from build123d import *

# Parameters (mm, degrees)
SKETCH_1_R          = 4.9999999999999964
EXTRUDE_1_DEPTH     = 18
SKETCH_2_R          = 5
EXTRUDE_2_DEPTH     = 8
FILLET_2_R          = 2
EXTRUDE_4_DEPTH     = 11.3
SKETCH_8_W          = 3.000000000000001
SKETCH_8_H          = 6.0000000000000036
CUT_EXTRUDE_3_DEPTH = 20
SKETCH_9_R          = 2.250000000000002
CUT_EXTRUDE_4_DEPTH = 78.37023084919184
FILLET_1_R          = 1
EXTRUDE_5_DEPTH     = 8
FILLET_3_R          = 2
EXTRUDE_6_DEPTH     = 11.3
FILLET_4_R          = 0.7
CHAMFER_2_SIZE      = 0.7
CUT_EXTRUDE_5_REACH = 123.985
CUT_EXTRUDE_6_DEPTH = 96.67513972142032


# Read off the part's stored shape, not the designer's step: 镜向1
with BuildPart() as part:
    # 草图1 → 凸台-拉伸1 (new body)
    with BuildSketch(Plane.XY):
        with BuildLine():
            Line((61.00000000000003, -13.176914536239765), (43, 17.999999999999996))
            Line((43, 17.999999999999996), (0, 18))
            ThreePointArc((0, 18), (-18, 2.2e-15), (0, -18))
            Line((0, -18), (43, -17.999999999999996))
            ThreePointArc((43, -17.999999999999996), (52.31748562369077, -16.77332974640645), (61.00000000000003, -13.176914536239765))
        make_face()
        with Locations((29.77, 0)):
            Circle(SKETCH_1_R, mode=Mode.SUBTRACT)
    extrude(amount=EXTRUDE_1_DEPTH)

    # 草图2 → 凸台-拉伸2 (add)
    with BuildSketch(Plane.XY.offset(18)):
        with BuildLine():
            Line((8.951308150188659, -4.435), (20.807256279464415, -4.435))
            ThreePointArc((20.807256279464415, -4.434999999999999), (19.769999999999996, 4.4e-16), (20.807256279464415, 4.435))
            Line((20.807256279464415, 4.435), (8.951308150188659, 4.435))
            ThreePointArc((8.951308150188659, 4.434999999999999), (9.989751878782268, -6.7e-16), (8.951308150188659, -4.435))
        make_face()
        Circle(SKETCH_2_R)
    extrude(amount=EXTRUDE_2_DEPTH)

    # 圆角2
    fillet_2_edges = [part.edges().sort_by_distance(p)[0] for p in [
        (20.807256279464415, -4.434999999999999, 22),
        (20.807256279464415, 4.434999999999999, 22),
        (8.951308150188659, 4.434999999999999, 22),
        (8.951308150188659, -4.434999999999999, 22),
    ]]
    fillet(fillet_2_edges, radius=FILLET_2_R)

    # 草图7 → 凸台-拉伸4 (add)
    with BuildSketch(Plane(origin=(33.99999999999993, 33.588457268120045, 0), x_dir=(0, 0, -1), z_dir=(-0.866025403784438, -0.5000000000000009, 0))):
        Polygon((-5.599999999999984, 54.00000000000014), (-12.400000000000015, 54.00000000000014), (-12.400000000000004, 18.00000000000018), (-5.599999999999972, 18.00000000000019), align=None)
        Polygon((-2.9999999999999973, 33.70000000000016), (-1.041e-14, 33.70000000000016), (-1.041e-14, 38.30000000000017), (-2.9999999999999956, 38.30000000000017), align=None)
        Polygon((-15.000000000000004, 38.30000000000017), (-17.99999999999999, 38.30000000000017), (-17.99999999999999, 33.70000000000016), (-15.000000000000002, 33.70000000000016), align=None)
    extrude(amount=-EXTRUDE_4_DEPTH)

    # 草图8 → 切除-拉伸3 (cut)
    with BuildSketch(Plane(origin=(49.8303156968241, 28.769546181365495, -2.936e-14), x_dir=(-5.4e-16, -3.2e-16, 1), z_dir=(0.866025403784438, 0.500000000000001, 0))):
        with Locations((8.99999999999995, 23.911542731880154)):
            Rectangle(SKETCH_8_W, SKETCH_8_H)
    extrude(amount=-CUT_EXTRUDE_3_DEPTH, mode=Mode.SUBTRACT)

    # 草图9 → 切除-拉伸4 (cut, through all)
    with BuildSketch(Plane(origin=(-8.8e-16, 1.52e-15, 5.59999999999997), x_dir=(-1, 0, -1e-16), z_dir=(1e-16, -1.7e-16, -1))):
        with Locations(Location((-60.946152422706646, -1.0836477965031495, 0), (0, 0, 90))):
            Circle(SKETCH_9_R)
        with Locations(Location((-53.44615242270663, 11.90673326026341, 0), (0, 0, 90))):
            Circle(SKETCH_9_R)
    extrude(amount=-CUT_EXTRUDE_4_DEPTH, mode=Mode.SUBTRACT)

    # 圆角1
    fillet_1_edges = [part.edges().sort_by_distance(p)[0] for p in [
        (54.62583302491982, 0.4634665205268087, 10.499999999999913),
        (51.625833024919814, 5.659618943233441, 10.499999999999913),
        (51.625833024919814, 5.659618943233441, 7.499999999999914),
        (54.62583302491982, 0.4634665205268087, 7.499999999999914),
        (55.74304353138211, 7.2284011605843475, 17.99999999999999),
        (58.043043531382125, 3.244684303175926, 17.99999999999999),
        (58.043043531382125, 3.244684303175926, 15.000000000000004),
        (55.74304353138211, 7.2284011605843475, 15.000000000000002),
        (55.74304353138211, 7.2284011605843475, 2.9999999999999973),
        (58.043043531382125, 3.244684303175926, 2.9999999999999956),
        (58.043043531382125, 3.244684303175926, 1.041e-14),
        (55.74304353138211, 7.2284011605843475, 1.041e-14),
    ]]
    fillet(fillet_1_edges, radius=FILLET_1_R)

    # 草图10 → 凸台-拉伸5 (add)
    with BuildSketch(Plane.XY.offset(18)):
        with BuildLine():
            Line((29.77, -10), (-14.966629547095765, -10))
            ThreePointArc((-14.966629547095765, -10), (-8.48528137423857, -15.874507866387544), (0, -18.000000000000004))
            Line((0, -18.000000000000004), (43, -17.999999999999996))
            ThreePointArc((43, -17.999999999999996), (52.31748562369077, -16.77332974640645), (61.00000000000003, -13.176914536239769))
            Line((61.00000000000003, -13.176914536239769), (43, 17.999999999999996))
            Line((43, 17.999999999999996), (0, 18.000000000000004))
            ThreePointArc((0, 18.000000000000004), (-8.485281374238571, 15.874507866387546), (-14.966629547095765, 10))
            Line((-14.966629547095765, 10), (29.77, 10))
            ThreePointArc((29.77, 10), (39.769999999999996, 0), (29.77, -10))
        make_face()
    extrude(amount=EXTRUDE_5_DEPTH)

    # 圆角3
    fillet_3_edges = [part.edges().sort_by_distance(p)[0] for p in [
        (-14.966629547095767, 10, 22),
        (-14.966629547095767, -10.000000000000002, 22),
    ]]
    fillet(fillet_3_edges, radius=FILLET_3_R)

    # 草图11 → 凸台-拉伸6 (add)
    with BuildSketch(Plane(origin=(49.8303156968241, 28.769546181365495, -2.936e-14), x_dir=(5.8e-16, 2.6e-16, -1), z_dir=(0.866025403784438, 0.500000000000001, 0))):
        Polygon((-12.400000000000041, -39.51154273188015), (-13.999999999999961, -39.51154273188015), (-13.999999999999966, -41.91154273188013), (-12.400000000000041, -41.91154273188013), align=None)
        Polygon((-3.999999999999961, -39.51154273188015), (-5.6000000000000085, -39.51154273188015), (-5.60000000000001, -41.91154273188014), (-3.99999999999997, -41.91154273188013), align=None)
        Polygon((-5.600000000000001, -5.911542731880182), (-5.600000000000002, -8.31154273188016), (-3.999999999999961, -8.31154273188016), (-3.999999999999969, -5.911542731880172), align=None)
        Polygon((-13.999999999999966, -5.911542731880174), (-13.999999999999966, -8.31154273188016), (-12.400000000000034, -8.31154273188016), (-12.400000000000034, -5.911542731880178), align=None)
    extrude(amount=-EXTRUDE_6_DEPTH)

    # 圆角4
    fillet_4_edges = [part.edges().sort_by_distance(p)[0] for p in [
        (64.69304353138213, -8.273453567157098, 13.999999999999932),
        (64.69304353138213, -8.273453567157091, 12.40000000000001),
        (65.89304353138213, -10.35191453623974, 13.999999999999936),
        (64.69304353138213, -8.273453567157091, 5.599999999999978),
        (64.69304353138213, -8.273453567157091, 3.9999999999999343),
        (65.89304353138213, -10.351914536239732, 3.999999999999939),
        (47.89304353138211, 20.825000000000003, 3.999999999999937),
        (49.09304353138211, 18.74653903091736, 3.999999999999932),
        (49.09304353138211, 18.74653903091736, 5.5999999999999694),
        (49.09304353138211, 18.746539030917358, 13.99999999999993),
        (49.09304353138211, 18.746539030917358, 12.4),
        (47.89304353138211, 20.825, 13.999999999999932),
    ]]
    fillet(fillet_4_edges, radius=FILLET_4_R)

    # 倒角2
    chamfer_2_edges = [part.edges().sort_by_distance(p)[0] for p in [
        (53.986087062764184, 21.571539030917368, 4.799999999999956),
        (61.7860870627642, 8.061542731880138, 12.40000000000001),
        (69.58608706276421, -5.448453567157085, 13.199999999999976),
        (70.1860870627642, -6.4876840516984196, 13.999999999999938),
        (70.78608706276421, -7.52691453623973, 8.99999999999994),
        (70.1860870627642, -6.487684051698405, 3.999999999999942),
        (69.58608706276421, -5.448453567157085, 4.799999999999963),
        (61.786087062764196, 8.061542731880149, 5.599999999999977),
        (53.38608706276419, 22.61076951545869, 3.99999999999994),
        (52.78608706276419, 23.650000000000006, 8.99999999999994),
        (53.38608706276418, 22.610769515458685, 13.999999999999936),
        (53.986087062764184, 21.571539030917364, 13.199999999999969),
        (70.6835744361795, -7.349357458577688, 4.205025253169361),
        (70.6835744361795, -7.349357458577694, 13.794974746830517),
        (52.88859968934889, 23.47244292233795, 13.79497474683052),
        (52.888599689348894, 23.472442922337958, 4.205025253169356),
        (69.6885996893489, -5.626010644819133, 4.20502525316936),
        (69.6885996893489, -5.62601064481914, 13.79497474683052),
        (53.883574436179465, 21.749096108579412, 13.794974746830519),
        (53.88357443617947, 21.74909610857942, 4.205025253169357),
        (54.0885996893489, 21.393981953255317, 5.394974746830557),
        (54.08859968934889, 21.393981953255313, 12.60502525316942),
        (69.4835744361795, -5.27089648949504, 12.60502525316943),
        (69.48357443617951, -5.270896489495035, 5.394974746830568),
    ]]
    chamfer(chamfer_2_edges, length=CHAMFER_2_SIZE)

    # 切除-拉伸5: up to this face of the body (flat: up to its plane)
    cut_extrude_5_end = Plane(part.part.faces().sort_by_distance((47.58993464, 20.65, 9))[0])
    # 草图12 → 切除-拉伸5 (cut, up to the picked face)
    with BuildSketch(Plane(origin=(98.23909236273093, 8.323085463760323, 0), x_dir=(-0.866025403784438, -0.500000000000001, 0), z_dir=(-0.500000000000001, 0.866025403784438, 0)), mode=Mode.PRIVATE) as cut_extrude_5_sk1:
        Polygon((31.700000000000067, 12.799999999999999), (31.700000000000067, 13.999999999999998), (32.90000000000007, 13.999999999999996), align=None)
    cut_extrude_5_tool1 = split(extrude(cut_extrude_5_sk1.sketch, amount=CUT_EXTRUDE_5_REACH, mode=Mode.PRIVATE), bisect_by=cut_extrude_5_end, keep=Keep.BOTH, mode=Mode.PRIVATE)
    # 草图12 → 切除-拉伸5 (cut, up to the picked face)
    with BuildSketch(Plane(origin=(98.23909236273093, 8.323085463760323, 0), x_dir=(-0.866025403784438, -0.500000000000001, 0), z_dir=(-0.500000000000001, 0.866025403784438, 0)), mode=Mode.PRIVATE) as cut_extrude_5_sk2:
        Polygon((31.700000000000067, 4.0000000000000036), (32.90000000000007, 4.000000000000005), (31.700000000000067, 5.200000000000003), align=None)
    cut_extrude_5_tool2 = split(extrude(cut_extrude_5_sk2.sketch, amount=CUT_EXTRUDE_5_REACH, mode=Mode.PRIVATE), bisect_by=cut_extrude_5_end, keep=Keep.BOTH, mode=Mode.PRIVATE)
    add(cut_extrude_5_tool1.solids().sort_by(Axis((70.439677, -7.726915, 13.6), (-0.500000000000001, 0.866025403784438, 0)))[0], mode=Mode.SUBTRACT)
    add(cut_extrude_5_tool2.solids().sort_by(Axis((70.439677, -7.726915, 4.4), (-0.500000000000001, 0.866025403784438, 0)))[0], mode=Mode.SUBTRACT)

    # 镜向1: part across plane


with BuildPart() as part_1:
    add(part.part)
    add(part.part.mirror(Plane(origin=(0, -18, 18), x_dir=(0, 0, 1), z_dir=(-8e-17, 1, 0))))

    # 草图13 → 切除-拉伸6 (cut, through all)
    with BuildSketch(Plane.XY.offset(26)):
        Polygon((-3.31e-15, -17.999999999999996), (43, -17.999999999999996), (87.8218201095251, -17.999999999999996), (87.8218201095251, 39.78196622179553), (-28.896212069890126, 39.78196622179553), (-28.896212069890126, -17.999999999999996), align=None)
    extrude(amount=-CUT_EXTRUDE_6_DEPTH, mode=Mode.SUBTRACT)


solid = part_1.part
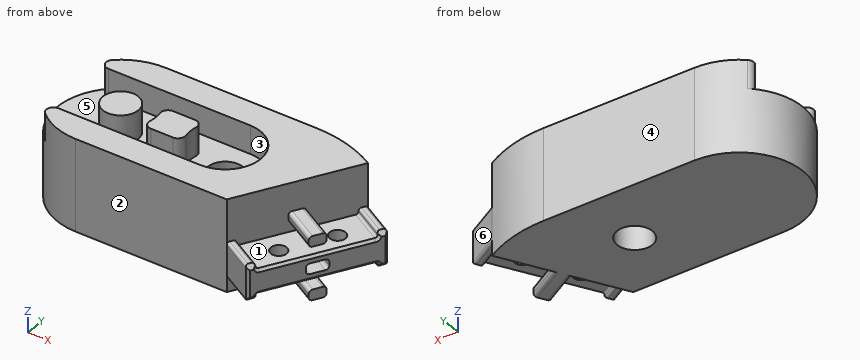
Model file for the job. Use its own axes, mm. Face numbers are marked on the shaded views. A direction names the side the tool comes from. Round coordinates to 2 decimals unless told otherwise and drop trailing zeros. Loops run counter-clockwise (first coordinate to the right, second up) from the corner with the lowest first, then second, coordinate; pieces in that order, holes last. Notation, with made-up numbers: (88, -16.75) - (122, -16.75) arc R21 cw to (122, 3.25) - close; hole circle Ø10 at (-29.5, 42.25). An arc over 180 degrees is marked (long way). Write each question's results on one line, items separated by ' | '.
(1) Saw through at C-C, the plane x = -3. List the corners of the cut face in (y, z), then the cut area to 3 significant figures.
Answer below:
outline: (-53.75, 0) - (-18.25, 0) - (-18.25, 26) - (-26, 26) - (-26, 18) - (-32, 18) - (-32, 26) - (-40, 26) - (-40, 18) - (-46, 18) - (-46, 26) - (-53.75, 26) - close | area: 827 mm^2
(2) Saw through at B-B, the plane z = 20. List the corners of the cut face in (x, y) (1 decimal).
Answer below:
outline: (-11.9, -49.5) arc R18 ccw to (0, -54) - (43, -54) - (61, -22.8) arc R36 ccw to (43, -18) - (0, -18) arc R18 ccw to (-11.9, -22.5) arc R2 ccw to (-10.6, -26) - (29.8, -26) arc R10 cw to (29.8, -46) - (-10.6, -46) arc R2 ccw to start; circle Ø10 at (0, -36); (9.8, -38) arc R2 ccw to (11.7, -40.4) - (18, -40.4) arc R2 ccw to (20, -38) arc R10 cw to (20, -34) arc R2 ccw to (18, -31.6) - (11.7, -31.6) arc R2 ccw to (9.8, -34) arc R10 cw to start
(3) Pin check, flat tips, straight feed: pin 1 (4 mm diameter, centred on y = -45, z = 4, fed in from -X); pin 2 (1.8 mm diameter, centred on x = 63.5, y = -27.5, fed in from +Z); pin 3 (16 mm diameter, centred on x = 29.77, y = -36, fed in from +Z). Stop position of each tip, or through.
Answer below:
pin 1: stops at x = -16.58 | pin 2: stops at z = 13.97 | pin 3: stops at z = 18
(4) 3-axis set-ups, long thin cutter, end or side, ignore diameter. For the marked faces 1, 2 and 3: which of +Z, -Z, +X, -X, +Y, -Y reach the whole face in a straight line?
Answer below:
face 1: none | face 2: +Z, -Z, -X, -Y | face 3: +Z
(5) Mould opens along X. For the marked faces 4, 5 and 6 say: released by +X, released by -X, zero draft, split by the parting line, or undercut.
Answer below:
face 4: zero draft | face 5: undercut | face 6: released by +X
(6) Wall check: L1, parallel to Y at x = 29.77, z = 13; L2, parallel to Z at x = 49, y = -36; L3, parallel to Z at x = 3.5, y = -29. Give the ranges that are in metal, low to high.
Answer below:
L1: y = -54 to -41, -31 to -18 | L2: z = 0 to 7.5, 10.5 to 26 | L3: z = 0 to 18
(7) Saw through at A-A, the plane x = 16.5. List the corners of the cut face in (y, z) (3 decimals), then the cut area to 3 significant figures.
Answer below:
outline: (-54, 0) - (-18, 0) - (-18, 26) - (-26, 26) - (-26, 18) - (-31.565, 18) - (-31.565, 26) - (-40.435, 26) - (-40.435, 18) - (-46, 18) - (-46, 26) - (-54, 26) - close | area: 847 mm^2
